Autodesk Inventor part; units mm, degrees
ref_plane "YZ Plane" through (0, 0, 0) normal (1, 0, 0) x (0, 1, 0)
ref_plane "XZ Plane" through (0, 0, 0) normal (0, 1, 0) x (-1, 0, 0)
ref_plane "XY Plane" through (0, 0, 0) normal (0, 0, 1) x (1, 0, 0)
sketch "Sketch2" plane through (0, 0, 0) normal (0, 0, 1) x (1, 0, 0)
  line L0 (-53, -88.9) -> (53, -88.9)
  line L1 (53, -88.9) -> (53, 88.9)
  line L2 (53, 88.9) -> (-53, 88.9)
  line L3 (-53, 88.9) -> (-53, -88.9)
  line L4 (-53, -88.9) -> (53, 88.9) construction
  line L5 (53, -88.9) -> (-53, 88.9) construction
  point P0 (0, 0)
  dimension "d0" = 106
  dimension "d1" = 177.8
extrude "Extrusion1" add sketch "Sketch2" against normal blind 6.35
sketch "Sketch5" plane through (0, 0, 0) normal (0, 0, 1) x (1, 0, 0)
  circle A0 centre (0, 0) radius 11.1125
  dimension "d26" = 22.225
extrude "CenterHole" cut sketch "Sketch5" against normal through all
sketch "Sketch6" plane through (0, 0, 0) normal (0, 0, 1) x (1, 0, 0)
  line L0 (-53, 88.9) -> (-53, -88.9)
  line L1 (53, -88.9) -> (53, 88.9)
  line L2 (-53, -88.9) -> (-53, 88.9) construction
  line L3 (-53, 82.4) -> (53, 82.4) construction
  line L4 (53, 88.9) -> (-53, 88.9) construction
  point P0 (0, 0)
  point P1 (0, 82.4)
  point P2 (123.3454, 23.3667)
  point P3 (-25, 82.4)
  point P4 (25, 82.4)
  dimension "d29" = 6.5
  dimension "d30" = 25
  dimension "d31" = 25
hole "TopThreeHoles" at (0, 82.4, 0) at (123.3454, 23.3667, 0) at (-25, 82.4, 0) at (25, 82.4, 0) direction (0, 0, -1) diameter 2.6416 end through all
sketch "Sketch7" plane through (0, 0, 0) normal (0, 0, 1) x (1, 0, 0)
  line L0 (53, -88.9) -> (53, 88.9)
  line L1 (-53, 88.9) -> (-53, -88.9)
  line L2 (-53, -38.1) -> (53, -38.1) construction
  line L3 (53, 88.9) -> (53, -88.9)
  line L4 (53, 88.9) -> (-53, 88.9) construction
  point P0 (0, 0)
  point P1 (-48, -38.1)
  point P2 (48, -38.1)
  dimension "d39" = 127
  dimension "d40" = 5
  dimension "d41" = 5
hole "BottomTwoHoles" at (-48, -38.1, 0) at (48, -38.1, 0) direction (0, 0, -1) diameter 2.6416 end through all
fillet "Fillet1" radius 1.5875 4 edges at (53, 88.9, -3.175) (-53, 88.9, -3.175) (53, -88.9, -3.175) (-53, -88.9, -3.175)
sketch "Sketch8" plane through (0, 0, 0) normal (0, 0, 1) x (1, 0, 0)
  line L0 (0, 0) -> (-53, 53) construction
  line L1 (-53, 87.3125) -> (-53, -87.3125) construction
  line L2 (-38.0224, 38.0224) -> (-29.3295, 29.3295) construction
  line L3 (-40.4112, 35.6337) -> (-31.7183, 26.9408)
  line L4 (-26.9408, 31.7183) -> (-35.6337, 40.4112)
  arc A0 (-35.6337, 40.4112) -> (-40.4112, 35.6337) centre (-38.0224, 38.0224) ccw
  arc A1 (-31.7183, 26.9408) -> (-26.9408, 31.7183) centre (-29.3295, 29.3295) ccw
  point P0 (-33.676, 33.676)
  dimension "d50" = 45
  dimension "d51" = 6.7564
  dimension "d53" = 19.05
  dimension "d59" = 3.3782
  dimension "d60" = 41.4782
extrude "SlotForScrews" cut sketch "Sketch8" against normal through all
pattern_circular "Circular Pattern1" count 4 over 360 about axis through (0, 0, -10) along (0, 0, 1) of "SlotForScrews"
properties part number "properySideGateGasket"
For this review, take the finished solid that the model builds, in its own axes (mm). A direction names the side the tool comes from. Coordinates: 2 decimals unless noted, no trailing zeros. Order: outer loops, then holes, each group sorted by start corner. A loop starts at its lowest first (then second) coordinate and runs counter-clockwise, first axis right, second up. Notation, with made-up numbers: (-32.5, 81.5) - (-11.5, 81.5) arc R21 ccw to (-11.5, 88.5) - close; hole circle Ø1 at (21, -3). An arc over 180 degrees is marked (long way). Answer as a JSON object with one key per item and string values. Group by question number.
1. We need section A-A on x = -4. State the section outline as (y, z) points.
2. For probe 1 along X at (y, z) = (82.4, -4); probe 2 along Y at (x, z) = (-25, -4.5); probe 3 along Y at (x, z) = (-38.5, -4), list the stretches that pass through material, from the lowest coordinate up.
3. The part is to be moulded in two halves that separate along X. For faces 3 (the flat face through (53, -1, -3)), 4 (the flat face through (-13, 1, 0)), 5 (the cylindrical face through (10.6, 3.34, -3.13)), say which applies: pulls with the +X half, pulls with the -X half, needs draft (parallel to the pull), parting line crosses it, or undercut.
4. We need section B-B on z = -2.25. Give the number of separate pieces and of enclosed holes in the cut face, then the cut area to 3 significant figures.
5. For faces 1 (the flat face through (-1, -88.9, -3)), 2 (the flat face through (-36.13, 31.35, -3.13)), list the 3-axis set-ups (+Z, -Z, +X, -X, +Y, -Y) from which the entire face can be reached by the end or side of a thin tool; tool diameter is ignored.
Final values:
{
 "1": {"outline": "(-88.9, -6.35) - (-10.37, -6.35) - (-10.37, 0) - (-88.9, 0) - close; (10.37, -6.35) - (88.9, -6.35) - (88.9, 0) - (10.37, 0) - close"},
 "2": {"probe 1": "-53 to -26.32, -23.68 to -1.32, 1.32 to 23.68, 26.32 to 53", "probe 2": "-88.9 to 81.08, 83.72 to 88.9", "probe 3": "-88.9 to -41.37, -33.72 to 33.72, 41.37 to 88.9"},
 "3": {"face 3": "pulls with the +X half", "face 4": "needs draft", "face 5": "undercut"},
 "4": {"separate pieces": "1", "enclosed holes": "10", "area": "18,000 mm²"},
 "5": {"face 1": "+Z, -Z, +X, -X, -Y", "face 2": "+Z, -Z"}
}
